```python
from build123d import *

# Parameters (mm, degrees)
SKETCH_1_R      = 5.5
EXTRUDE_1_DEPTH = 34.2
SKETCH_2_R      = 8
EXTRUDE_2_DEPTH = 5
SKETCH_3_R      = 7.5
EXTRUDE_3_DEPTH = 5
SKETCH_5_R      = 5
EXTRUDE_4_DEPTH = 5


with BuildPart() as part:
    # ｽｹｯﾁ1 → ﾎﾞｽ - 押し出し1 (new body)
    with BuildSketch(Plane.XY):
        Circle(SKETCH_1_R)
    extrude(amount=EXTRUDE_1_DEPTH)

    # ｽｹｯﾁ2 → ﾎﾞｽ - 押し出し2 (add)
    with BuildSketch(Plane.XY.offset(34.2)):
        Circle(SKETCH_2_R)
    extrude(amount=-EXTRUDE_2_DEPTH)

    # ｽｹｯﾁ3 → ﾎﾞｽ - 押し出し3 (add)
    with BuildSketch(Plane.XY.offset(34.2)):
        Circle(SKETCH_3_R)
    extrude(amount=EXTRUDE_3_DEPTH)

    # ｽｹｯﾁ5 → ﾎﾞｽ - 押し出し4 (add)
    with BuildSketch(Plane(origin=(0, 0, 0), x_dir=(-1, 0, 0), z_dir=(0, 0, -1))):
        Circle(SKETCH_5_R)
    extrude(amount=EXTRUDE_4_DEPTH)


solid = part.part
```
Check sheet for the modelled part. Datum: model origin and axes. Units: mm. A direction names the side the tool comes from. Give positions to 0.01 mm unless a question says otherwise; leave off trailing zeros. Loops run counter-clockwise (first coordinate to the right, second up) from the corner with the lowest first, then second, coordinate; pieces in that order, holes last. Notation, with made-up numbers: (69.5, 86) - (107.5, 86) arc R18 ccw to (107.5, 90) - close; hole circle Ø8 at (37.5, 87.5). An arc over 180 degrees is marked (long way). One line per question, with ' | ' between items. Start each with the question number.
1. Material ranges on line 1 along Y through (x, z) = (0, 17.5); line 2 along Z through (x, y) = (-1, 5.5); line 3 along X through (y, z) = (2, 17.5), recorded low to high. Write a range as [from, to].
2. Cross-section at D-D, the plane z = 11. Enter the section's corners in (x, y).
3. Cross-section at C-C, the plane z = 32. Enter the section's corners in (x, y).
4. Draft check along X on faces 1 (the flat face through (1.7, 5.4, 29.2)), 2 (the cylindrical face through (-7.493, 0.33, 36.665)). Enter one of: released by +X, released by -X, zero draft, split by the parting line, or undercut.
5. Cross-section at A-A, the plane x = 0. Enter the section's corners in (y, z).
6. Gauge pin test, flat ends, axial feed: pin 1 Ø8 at (y, z) = (2, 5.5) entering from +X; pin 2 Ø1.5 at (x, z) = (5, 8.5) entering from +Y; pin 3 Ø3 at (y, z) = (6, 3.5) entering from +X. Record the tip position at first contact, or that the pin passes through.
7. Set-up check for faces 3 (the flat face through (5, -6, 34.2)), 4 (the cylindrical face through (-1.19, -5.37, 14.4)), 5 (the flat face through (0, 0, 39.2)): record each of +Z, -Z, +X, -X, +Y, -Y from which the full face is reachable in a straight line by a thin tool's end or side.
Check result:
1) line 1: y = [-5.5, 5.5] | line 2: z = [29.2, 39.2] | line 3: x = [-5.12, 5.12]
2) outline: circle Ø11 at (0, 0)
3) outline: circle Ø16 at (0, 0)
4) face 1: zero draft | face 2: split by the parting line
5) outline: (-8, 29.2) - (-5.5, 29.2) - (-5.5, 0) - (-5, 0) - (-5, -5) - (5, -5) - (5, 0) - (5.5, 0) - (5.5, 29.2) - (8, 29.2) - (8, 34.2) - (7.5, 34.2) - (7.5, 39.2) - (-7.5, 39.2) - (-7.5, 34.2) - (-8, 34.2) - close
6) pin 1: stops at x = 5.5 | pin 2: stops at y = 3.49 | pin 3: stops at x = 3.16
7) face 3: +Z | face 4: -Z | face 5: +Z, +X, -X, +Y, -Y
